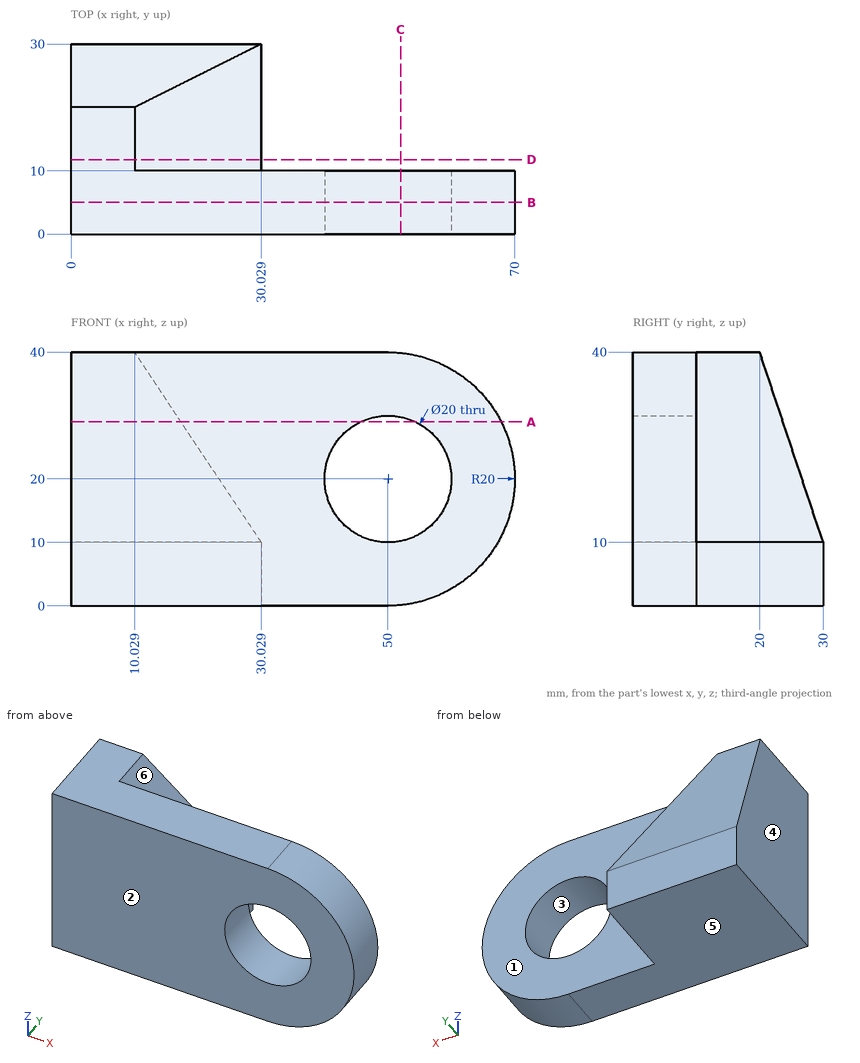
Input: dimensioned drawing with shaded views. Units: mm. Origin: part minimum x, y, z. A direction names the side the tool comes from. Give positions to 0.01 mm unless a question says otherwise; leave off trailing zeros. Loops run counter-clockwise (first coordinate to the right, second up) from the corner with the lowest first, then second, coordinate; pieces in that order, holes last. Notation, with made-up numbers: (59, 2) -> (71, 2) arc R22 ccw to (71, 26) -> close; hole circle Ø2 at (-8.5, 30.25). An arc over 180 degrees is marked (long way). Return JSON: item names as keys, results as strings.
Item 1: Section D-D, the plane y = 11.75. Output: boundary loops of the cut face in (x, z).
Filled in:
{"outline": "(0, 0) -> (30.03, 0) -> (30.03, 10) -> (10.03, 40) -> (0, 40) -> close"}
Item 2: Section C-C, the plane x = 52. Output: boundary loops of the cut face in (y, z).
Filled in:
{"outline": "(0, 0.1) -> (10, 0.1) -> (10, 10.2) -> (0, 10.2) -> close; (0, 29.8) -> (10, 29.8) -> (10, 39.9) -> (0, 39.9) -> close"}
Item 3: Line query: line 1 (X direction, y = 7.75, z = 20); line 2 (Y direction, x = 44, z = 37); line 3 (X direction, y = 23.5, z = 6.5). Output: solid intervals per line, ascending.
Filled in:
{"line 1": "0 to 40, 60 to 70", "line 2": "0 to 10", "line 3": "0 to 30.03"}
Item 4: Mould query, pull axis Z, two halves, no side actions, for the marked faces 3, 4, 5 and 6. Classes: released by +Z, released by -Z, zero draft, split by the parting line, or undercut.
Filled in:
{"face 3": "undercut", "face 4": "zero draft", "face 5": "released by -Z", "face 6": "released by +Z"}
Item 5: Access query for the marked faces 1 and 2. Directions: +Z, -Z, +X, -X, +Y, -Y. A direction counts if a zero-diameter tool reaches every point of the face in a straight line with its end or side. Return the directions, or none.
Filled in:
{"face 1": "+Z, +X, +Y", "face 2": "+Z, -Z, +X, -X, -Y"}
Item 6: Section A-A, the plane z = 29. Output: boundary loops of the cut face in (x, y), plus the area to 3 significant figures.
Filled in:
{"outline": "(0, 0) -> (45.64, 0) -> (45.64, 10) -> (17.36, 10) -> (17.36, 23.67) -> (0, 23.67) -> close; (54.36, 0) -> (67.86, 0) -> (67.86, 10) -> (54.36, 10) -> close", "area": "829 mm^2"}
Item 7: Section B-B, the plane y = 5. Output: boundary loops of the cut face in (x, z).
Filled in:
{"outline": "(0, 0) -> (50, 0) arc R20 ccw to (50, 40) -> (0, 40) -> close; hole circle Ø20 at (50, 20)"}
Item 8: Pin query (flat end, axial travel): P1, Ø4, axis at x = 42.5, z = 29.5, coming from the +Y side; P2, Ø8, axis at y = 22.5, z = 3, coming from the +X side; P3, Ø12, axis at x = 50, z = 20, coming from the -Y side; P4, Ø1.5, axis at y = 17, z = 20, coming from the +X side. Return the tip coordinate at first contact, or that it passes through.
Filled in:
{"P1": "y = 10", "P2": "x = 30.03", "P3": "through", "P4": "x = 23.86"}
